from build123d import *

# Parameters (mm, degrees)
SKETCH1_R             = 17.5
BOSS_EXTRUDE1_DEPTH   = 1.5
SKETCH3_W             = 1
SKETCH3_H             = 1.5
BOSS_EXTRUDE3_DEPTH   = 0.5
BOSS_EXTRUDE4_START   = 3
SKETCH3_4_R           = 17.5
BOSS_EXTRUDE4_DEPTH   = 3
BOSS_EXTRUDE6_DEPTH   = 2.5
BODY_MOVE_COPY1_ANGLE = 90


with BuildPart() as part:
    # Sketch1 → Boss-Extrude1 (new body)
    with BuildSketch(Plane(origin=(0, 0, 0), x_dir=(1, 0, 0), z_dir=(0, 1, 0))):
        with Locations(Location((0, 0, 0), (0, 0, 270))):
            Circle(SKETCH1_R)
    extrude(amount=BOSS_EXTRUDE1_DEPTH)

    # Sketch3 → Boss-Extrude3 (add)
    with BuildSketch(Plane.XZ):
        with Locations((0, 15.75)):
            Rectangle(SKETCH3_W, SKETCH3_H)
    extrude(amount=BOSS_EXTRUDE3_DEPTH)

    # Sketch3<4> → Boss-Extrude4 (add)
    with BuildSketch(Plane.XZ.offset(BOSS_EXTRUDE4_START)):
        with Locations(Location((0, 0, 0), (0, 0, 270))):
            Circle(SKETCH3_4_R)
        with BuildLine():
            Line((-0.5, 16.5), (0.5, 16.5))
            Line((0.5, 16.5), (0.5, 16.492422502))
            ThreePointArc((0.5, 16.492422502), (0, -16.5), (-0.5, 16.492422502))
            Line((-0.5, 16.492422502), (-0.5, 16.5))
        make_face(mode=Mode.SUBTRACT)
    extrude(amount=-BOSS_EXTRUDE4_DEPTH)

    # Sketch4 → Boss-Extrude6 (add)
    with BuildSketch(Plane.XZ.offset(3)):
        with BuildLine():
            Line((-0.5, 16.5), (-0.5, 16.492422502))
            ThreePointArc((-0.5, 16.492422502), (-0.250028708, 16.498105517), (0, 16.5))
            Line((0, 16.5), (-0.5, 16.5))
        make_face()
        with BuildLine():
            Line((0.5, 16.5), (0, 16.5))
            ThreePointArc((0, 16.5), (0.250028708, 16.498105517), (0.5, 16.492422502))
            Line((0.5, 16.492422502), (0.5, 16.5))
        make_face()
    extrude(amount=-BOSS_EXTRUDE6_DEPTH)

    # Split2
    split(bisect_by=Plane(origin=(0, 0, 0), x_dir=(-1, 0, 0), z_dir=(0, 0, -1)), keep=Keep.BOTTOM)

    # Mirror1: part across plane


with BuildPart() as part_1:
    add(part.part)
    add(part.part.mirror(Plane(origin=(0, 0, 0), x_dir=(1, 0, 0), z_dir=(0, 0, -1))))


with BuildPart() as body_2:
    # Body-Move/Copy1: copy of part
    add(part_1.part.rotate(Axis((0, 0, 0), (0, 1, 0)), BODY_MOVE_COPY1_ANGLE))


with BuildPart() as part_2:
    add(part_1.part)

    # Combine1: union body 2
    add(body_2.part)


solid = part_2.part
Work out the finished part from the listing and answer in its coordinate system (mm). A direction names the side the tool comes from. Give positions to 0.01 mm unless a question says otherwise; leave off trailing zeros. Write each loop counter-clockwise with the first axis right and the second up, starting at its lowest first coordinate (ties: lowest second). Pieces come first, ordered by that corner, then holes. Notation, with made-up numbers: M -29.75,8 L 18.25,8 A23 ccw 18.25,41 Z; hole C 57.5,31 d5. An arc over 180 degrees is marked long. Answer as CSV lines item,"result".
Q1. A cutting plane is placed at C-C on z = -3. Write down the section's boundary in (x, y), plus the area to 3 significant figures.
A:
outline,"M -17.24,-3 L -16.22,-3 L -16.22,0 L 16.22,0 L 16.22,-3 L 17.24,-3 L 17.24,1.5 L -17.24,1.5 Z"
area,"57.8 mm²"
Q2. A cutting plane is placed at D-D on y = 0.8. Write down the section's boundary in (x, z).
A:
outline,"C 0,0 d35"
Q3. The mould has two halves that part along X. Classify faces 1 (the cylindrical face through (-13.887, -0.781, -10.648)), 2 (the flat face through (-16, -3, -5)), 3 (the flat face through (0, -0.5, 16)): +X half, -X half, draft (parallel to the pull), parting line (faces both ways), or undercut.
A:
face 1,"parting line"
face 2,"draft"
face 3,"undercut"
Q4. Find the intervals of material crossed by probe 1 along Y at (x, z) = (-6, 10); probe 2 along Z at (x, y) = (0, -2.7); probe 3 along Z at (x, y) = (-3.5, -1.85), in increasing order. Write a range as [from, to].
A:
probe 1,"y = [0, 1.5]"
probe 2,"z = [-17.5, -16.5], [16.5, 17.5]"
probe 3,"z = [-17.15, -16.12], [16.12, 17.15]"
Q5. A cutting plane is placed at B-B on x = -14. Write down the section's boundary in (y, z), plus the area to 3 significant figures.
A:
outline,"M -3,-10.5 L 1.5,-10.5 L 1.5,10.5 L -3,10.5 L -3,8.73 L 0,8.73 L 0,-8.73 L -3,-8.73 Z"
area,"42.1 mm²"
Q6. A tool of negligible diameter and unlimited length cuts with its end or side. For faces 4 (the flat face through (16, -0.5, 0)), 5 (the flat face through (0, 1.5, 0)), from which of +Z, -Z, +X, -X, +Y, -Y can it reach the whole face along a straight path? Write none if from no direction.
A:
face 4,"-Y"
face 5,"+Z, -Z, +X, -X, +Y"
Q7. Given P1, Ø2, axis at x = -2.5, y = 0.5, coming from the -Z side; P2, Ø2, axis at y = -1.5, z = -12, coming from the -X side; P3, Ø0.6, axis at y = 0, z = -16, coming from the -X side, each flat-ended and moving along its own axis, determine where each tip first touches the part or whether it passes through.
A:
P1,"stops at z = -17.44"
P2,"stops at x = -13.61"
P3,"stops at x = -7.73"
